```python
from build123d import *

# Parameters (mm, degrees)
BOSS_EXTRUDE1_DEPTH = 5
SKETCH4_R           = 1.5
CUT_EXTRUDE1_DEPTH  = 5


with BuildPart() as part:
    # Sketch3 → Boss-Extrude1 (new body)
    with BuildSketch(Plane.XY):
        with BuildLine():
            Line((-70, 15), (150, 15))
            ThreePointArc((150, 15), (165, 0), (150, -15))
            Line((150, -15), (-70, -15))
            ThreePointArc((-70, -15), (-85, 0), (-70, 15))
        make_face()
    extrude(amount=BOSS_EXTRUDE1_DEPTH)

    # Sketch4 → Cut-Extrude1 (cut)
    with BuildSketch(Plane(origin=(0, 0, 0), x_dir=(-1, 0, 0), z_dir=(0, 0, -1))):
        with Locations((-150, 0)):
            Circle(SKETCH4_R)
        Circle(SKETCH4_R)
        with Locations((70, 0)):
            Circle(SKETCH4_R)
    extrude(amount=-CUT_EXTRUDE1_DEPTH, mode=Mode.SUBTRACT)


solid = part.part
```
CAD build for the part. Positions are in the model's coordinates, mm. Coordinates: 2 decimals unless noted, no trailing zeros. Order: outer loops, then holes, each group sorted by start corner. A loop starts at its lowest first (then second) coordinate and runs counter-clockwise, first axis right, second up. Notation, with made-up numbers: (25, 40) - (66, 40) arc R23 ccw to (66, 56) - close; hole circle Ø6 at (63.25, 42). An arc over 180 degrees is marked (long way). Use a Markdown table: item, result. Add a question column.
(1) Saw through at A-A (z = 0.85). Give the cut face in (x, y).
(2) Saw through at B-B (y = -11). Give the cut face in (x, z).
(3) Flat gauge pins, fed straight in: pin 1 (2.5 mm diameter, centred on x = -70, y = 0, fed in from -Z); pin 2 (3 mm diameter, centred on y = -8.5, z = 1, fed in from +X); pin 3 (1.5 mm diameter, centred on x = 26, y = 1.5, fed in from -Z). Where does each tip first touch, or does it go through?
(4) Drill centre lines: line 1 along Y through (x, z) = (0, 1.2); line 2 along X through (y, z) = (-0.5, 1.15); line 3 along X through (y, z) = (1, 0.2). Where is each one in solid material? Low to high. Write a range as [from, to].
Solved:
| question | item | result |
|---|---|---|
| 1 | outline | (-70, -15) - (150, -15) arc R15 ccw to (150, 15) - (-70, 15) arc R15 ccw to start; hole circle Ø3 at (-70, 0); hole circle Ø3 at (0, 0); hole circle Ø3 at (150, 0) |
| 2 | outline | (-80.2, 0) - (160.2, 0) - (160.2, 5) - (-80.2, 5) - close |
| 3 | pin 1 | passes through |
| 3 | pin 2 | stops at x = 163.27 |
| 3 | pin 3 | stops at z = 0 |
| 4 | line 1 | y = [-15, -1.5], [1.5, 15] |
| 4 | line 2 | x = [-84.99, -71.41], [-68.59, -1.41], [1.41, 148.59], [151.41, 164.99] |
| 4 | line 3 | x = [-84.97, -71.12], [-68.88, -1.12], [1.12, 148.88], [151.12, 164.97] |
